Check sheet for the modelled part. Datum: model origin and axes. Units: mm. A direction names the side the tool comes from. Round coordinates to 2 decimals unless told otherwise and drop trailing zeros. Write each loop counter-clockwise with the first axis right and the second up, starting at its lowest first coordinate (ties: lowest second). Pieces come first, ordered by that corner, then holes. Notation, with made-up numbers: M -15,47.5 L 15,47.5 A27 ccw 15,67.5 Z; hole C -32.75,75 d5. An arc over 180 degrees is marked long. Answer in a Markdown table with one row per item.
Autodesk Inventor part; units mm, degrees
ref_plane "Start Plane" through (0, 0, 0) normal (1, 0, 0) x (0, 1, 0)
ref_plane "XZ Plane" through (0, 0, 0) normal (0, 1, 0) x (-1, 0, 0)
ref_plane "XY Plane" through (0, 0, 0) normal (0, 0, 1) x (1, 0, 0)
sketch "Main Sketch" plane through (0, 0, 0) normal (0, 0, 1) x (1, 0, 0)
  line L0 (0, 0) -> (130.7338, 0)
  line L1 (0, 0) -> (0, 7.9216)
  line L2 (0, 7.9216) -> (20.6375, 7.9216)
  line L3 (20.6375, 7.9216) -> (20.6375, 11.3284)
  line L4 (39.4335, 11.3284) -> (39.4335, 7.9216)
  line L5 (20.6375, 11.3284) -> (39.4335, 11.3284)
  line L6 (59.2963, 7.9216) -> (59.2963, 6.35)
  line L7 (39.4335, 7.9216) -> (59.2963, 7.9216)
  line L8 (130.7338, 6.35) -> (130.7338, 0)
  line L9 (59.2963, 6.35) -> (130.7338, 6.35)
  dimension "d3" = 15.8432
  dimension "d4" = 22.6568
  dimension "d5" = 15.8432
  dimension "d6" = 12.7
revolve "Revolution1" add sketch "Main Sketch" angle 360 about axis through (0, 0, 0) along (1, 0, 0)
chamfer "Chamfer1" distance 0.7937 angle 45 1 edges at (0, -7.9216, 0) measured on face at (13.7583, 7.8959, -0.6374)
chamfer "Chamfer2" distance 1.5875 angle 45 1 edges at (130.7338, -6.35, 0) measured on face at (106.9213, 6.2678, -1.0186)
thread "Thread1"
sketch "Sketch3" plane through (0, 0, 0) normal (0, 0, 1) x (1, 0, 0)
  arc A0 (67.6045, 7.4481) -> (80.2341, 7.4481) centre (73.9193, 7.4481) ccw
  line L0 (67.6045, 7.4481) -> (80.2341, 7.4481)
  line L1 (59.2963, -7.9216) -> (59.2963, 7.9216) construction
  point P0 (0, 0)
  dimension "d16" = 14.623
  dimension "d17" = 6.3148
extrude "Extrusion1" cut sketch "Sketch3" along normal mid plane 1.5875
sketch "Sketch4" plane through (39.4335, 0, 0) normal (1, 0, 0) x (0, 0, -1)
  arc A0 (-8.9345, 13.3715) -> (-7.4665, 8.514) centre (3.948, 14.6141) ccw
  arc A1 (-7.4665, 8.514) -> (-8.514, 7.4665) centre (0, 0) ccw
  arc A2 (-8.514, 7.4665) -> (-13.3715, 8.9345) centre (-14.6141, -3.948) ccw
  arc A3 (-13.3715, 8.9345) -> (-14.4233, 7.1128) centre (0, 0) ccw
  arc A4 (-14.4233, 7.1128) -> (-10.7232, 3.64) centre (-3.888, 14.6302) ccw
  arc A5 (-10.7232, 3.64) -> (-11.1066, 2.2092) centre (0, 0) ccw
  arc A6 (-11.1066, 2.2092) -> (-16.0473, 1.0518) centre (-10.6822, -10.7261) ccw
  arc A7 (-16.0473, 1.0518) -> (-16.0473, -1.0518) centre (0, 0) ccw
  arc A8 (-16.0473, -1.0518) -> (-11.1066, -2.2092) centre (-10.6822, 10.7261) ccw
  arc A9 (-11.1066, -2.2092) -> (-10.7232, -3.64) centre (0, 0) ccw
  arc A10 (-10.7232, -3.64) -> (-14.4233, -7.1128) centre (-3.888, -14.6302) ccw
  arc A11 (-14.4233, -7.1128) -> (-13.3715, -8.9345) centre (0, 0) ccw
  arc A12 (-13.3715, -8.9345) -> (-8.514, -7.4665) centre (-14.6141, 3.948) ccw
  arc A13 (-8.514, -7.4665) -> (-7.4665, -8.514) centre (0, 0) ccw
  arc A14 (-7.4665, -8.514) -> (-8.9345, -13.3715) centre (3.948, -14.6141) ccw
  arc A15 (-8.9345, -13.3715) -> (-7.1128, -14.4233) centre (0, 0) ccw
  arc A16 (-7.1128, -14.4233) -> (-3.64, -10.7232) centre (-14.6302, -3.888) ccw
  arc A17 (-3.64, -10.7232) -> (-2.2092, -11.1066) centre (0, 0) ccw
  arc A18 (-2.2092, -11.1066) -> (-1.0518, -16.0473) centre (10.7261, -10.6822) ccw
  arc A19 (-1.0518, -16.0473) -> (1.0518, -16.0473) centre (0, 0) ccw
  arc A20 (1.0518, -16.0473) -> (2.2092, -11.1066) centre (-10.7261, -10.6822) ccw
  arc A21 (2.2092, -11.1066) -> (3.64, -10.7232) centre (0, 0) ccw
  arc A22 (3.64, -10.7232) -> (7.1128, -14.4233) centre (14.6302, -3.888) ccw
  arc A23 (7.1128, -14.4233) -> (8.9345, -13.3715) centre (0, 0) ccw
  arc A24 (8.9345, -13.3715) -> (7.4665, -8.514) centre (-3.948, -14.6141) ccw
  arc A25 (7.4665, -8.514) -> (8.514, -7.4665) centre (0, 0) ccw
  arc A26 (8.514, -7.4665) -> (13.3715, -8.9345) centre (14.6141, 3.948) ccw
  arc A27 (13.3715, -8.9345) -> (14.4233, -7.1128) centre (0, 0) ccw
  arc A28 (14.4233, -7.1128) -> (10.7232, -3.64) centre (3.888, -14.6302) ccw
  arc A29 (10.7232, -3.64) -> (11.1066, -2.2092) centre (0, 0) ccw
  arc A30 (11.1066, -2.2092) -> (16.0473, -1.0518) centre (10.6822, 10.7261) ccw
  arc A31 (16.0473, -1.0518) -> (16.0473, 1.0518) centre (0, 0) ccw
  arc A32 (16.0473, 1.0518) -> (11.1066, 2.2092) centre (10.6822, -10.7261) ccw
  arc A33 (11.1066, 2.2092) -> (10.7232, 3.64) centre (0, 0) ccw
  arc A34 (10.7232, 3.64) -> (14.4233, 7.1128) centre (3.888, 14.6302) ccw
  arc A35 (14.4233, 7.1128) -> (13.3715, 8.9345) centre (0, 0) ccw
  arc A36 (13.3715, 8.9345) -> (8.514, 7.4665) centre (14.6141, -3.948) ccw
  arc A37 (8.514, 7.4665) -> (7.4665, 8.514) centre (0, 0) ccw
  arc A38 (7.4665, 8.514) -> (8.9345, 13.3715) centre (-3.948, 14.6141) ccw
  arc A39 (8.9345, 13.3715) -> (7.1128, 14.4233) centre (0, 0) ccw
  arc A40 (7.1128, 14.4233) -> (3.64, 10.7232) centre (14.6302, 3.888) ccw
  arc A41 (3.64, 10.7232) -> (2.2092, 11.1066) centre (0, 0) ccw
  arc A42 (2.2092, 11.1066) -> (1.0518, 16.0473) centre (-10.7261, 10.6822) ccw
  arc A43 (1.0518, 16.0473) -> (-1.0518, 16.0473) centre (0, 0) ccw
  arc A44 (-1.0518, 16.0473) -> (-2.2092, 11.1066) centre (10.7261, 10.6822) ccw
  arc A45 (-2.2092, 11.1066) -> (-3.64, 10.7232) centre (0, 0) ccw
  arc A46 (-3.64, 10.7232) -> (-7.1128, 14.4233) centre (-14.6302, 3.888) ccw
  arc A47 (-7.1128, 14.4233) -> (-8.9345, 13.3715) centre (0, 0) ccw
extrude "Extrusion2" add sketch "Sketch4" against normal up to surface (18.796 mm away)
properties part number "Shaft" material "Aluminum 6061"
1. Go/stop test with flat-tipped pins: pin 1 (1 mm diameter, centred on y = -7.5, z = 12, fed in from -X); pin 2 (10 mm diameter, centred on y = 8.5, z = -1.5, fed in from +X); pin 3 (1.5 mm diameter, centred on x = 27.5, z = 12.5, fed in from +Y); pin 4 (4 mm diameter, centred on x = 30, y = -8.5, fed in from -Z). Record where each tip stops, or that it passes through.
Found:
| item | result |
|---|---|
| pin 1 | stops at x = 20.64 |
| pin 2 | stops at x = 130.73 |
| pin 3 | stops at y = 8.92 |
| pin 4 | stops at z = -14.42 |
2. Scan lines: L1, parallel to X at y = 12.5, z = -7; L2, parallel to Y at x = 104.5, z = 0.5; L3, parallel to Y at x = 49, z = 4.5. Record each from-to range of solid material in increasing order.
Found:
| item | result |
|---|---|
| L1 | x = 20.64 to 39.43 |
| L2 | y = -6.33 to 6.33 |
| L3 | y = -6.52 to 6.52 |
3. Access from +Z, -Z, +X, -X, +Y, -Y to the whole of each face (thin tool, end or side, straight path). Record for faces 1 (the face through (30.167, 12.773, -5.219)), 2 (the face through (30.167, -12.773, 5.219)), 3 (the face through (74, 4, -0.794)).
Found:
| item | result |
|---|---|
| face 1 | +X, -X, +Y |
| face 2 | +X, -X, -Y |
| face 3 | +Y |
4. Section check A-A, the plane x = 49.5. Record the cut outline in (y, z).
Found:
| item | result |
|---|---|
| outline | C 0,0 d15.84 |
5. Section check B-B, the plane x = 87. Record the cut outline in (y, z).
Found:
| item | result |
|---|---|
| outline | C 0,0 d12.7 |
6. Draft check along Z on faces 4 (the face through (30.167, -8.452, 10.906)), 5 (the face through (59.296, 0, 6.5)), 6 (the face through (10.855, -1.717, -7.733)), 7 (the face through (30.17, 5.17, -12.72)). Enter one of: +Z half, -Z half, draft (parallel to the pull), parting line (faces both ways), or undercut.
Found:
| item | result |
|---|---|
| face 4 | undercut |
| face 5 | draft |
| face 6 | parting line |
| face 7 | -Z half |
